Here's the drawing with two shaded views (mm, measured from the low corner). I have some questions. A direction names the side the tool comes from. Give positions to 0.01 mm unless a question says otherwise; leave off trailing zeros. Write each loop counter-clockwise with the first axis right and the second up, starting at its lowest first coordinate (ties: lowest second). Pieces come first, ordered by that corner, then holes. Notation, with made-up numbers: (53.25, -30.75) - (106.25, -30.75) arc R21 ccw to (106.25, 5.25) - close; hole circle Ø8 at (89, 46.25). An arc over 180 degrees is marked (long way). Answer as a JSON object with one key per item and string values. Group by question number.
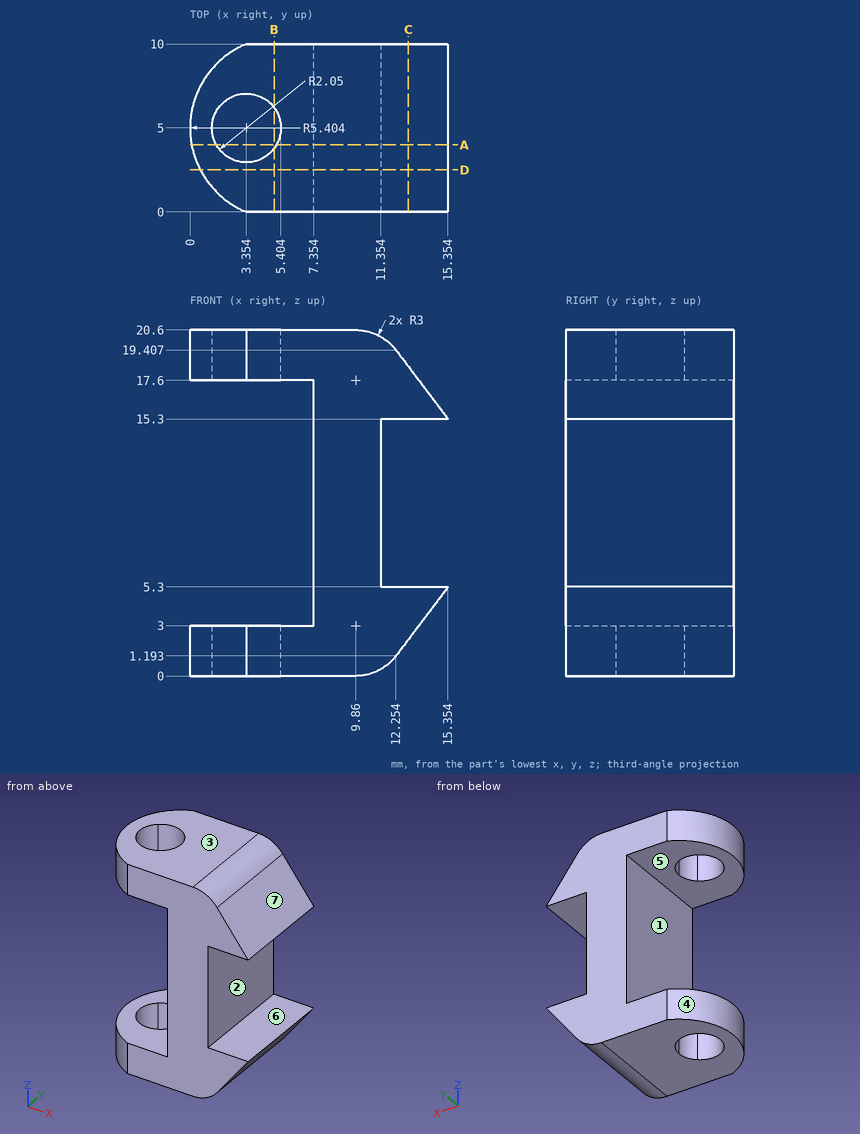
(1) I want a section at A-A, the plane y = 4. Please give me the cut outline in (x, z) (1 decimal).
(2) I want a section at C-C, the plane x = 13. Please give me the cut outline in (y, z).
(3) If we mould it in two halves opening along Z, with no side actions, what happens to the marked faces 4, 5, 6 and 7? For each: +Z half, -Z half, draft (parallel to the pull), parting line (faces both ways), or undercut.
(4) Will these pins go through, and if not, where does the flat tip stop? P1, Ø3, axis at y = 6, z = 10, coming from the +X side; P2, Ø1.2, axis at x = 13, y = 5, coming from the -Z side (1 decimal); P3, Ø3, axis at y = 7, z = 5.5, coming from the -X side.
(5) I need wall thicknesses on L1, parallel to Z at x = 2.75, y = 9; L2, parallel to Z at x = 12.75, y = 2.5; L3, parallel to Y at x = 4, z = 2.75 (1 decimal). Which ranges of each line are inside material? Lowest first, please.
(6) I want a section at B-B, the plane x = 5. Please give me the cut outline in (y, z).
(7) I want a section at D-D, the plane y = 2.5. Please give me the cut outline in (x, z) (1 decimal), and give its area (3 significant figures).
(8) For the marked faces 1, 2 and 3, which set-ups out of +Z, -Z, +X, -X, +Y, -Y let a thin tool reach every point of the face, with its end or its side?
Entries:
{
 "1": {"outline": "(0.1, 0) - (1.6, 0) - (1.6, 3) - (0.1, 3) - close; (0.1, 17.6) - (1.6, 17.6) - (1.6, 20.6) - (0.1, 20.6) - close; (5.1, 0) - (9.9, 0) arc R3 ccw to (12.3, 1.2) - (15.4, 5.3) - (11.4, 5.3) - (11.4, 15.3) - (15.4, 15.3) - (12.3, 19.4) arc R3 ccw to (9.9, 20.6) - (5.1, 20.6) - (5.1, 17.6) - (7.4, 17.6) - (7.4, 3) - (5.1, 3) - close"},
 "2": {"outline": "(0, 2.18) - (10, 2.18) - (10, 5.3) - (0, 5.3) - close; (0, 15.3) - (10, 15.3) - (10, 18.42) - (0, 18.42) - close"},
 "3": {"face 4": "draft", "face 5": "undercut", "face 6": "undercut", "face 7": "+Z half"},
 "4": {"P1": "x = 11.35", "P2": "z = 1.4", "P3": "x = 7.35"},
 "5": {"L1": "0 to 3, 17.6 to 20.6", "L2": "1.85 to 5.3, 15.3 to 18.75", "L3": "0 to 3.1, 6.9 to 10"},
 "6": {"outline": "(0, 0) - (3.78, 0) - (3.78, 3) - (0, 3) - close; (0, 17.6) - (3.78, 17.6) - (3.78, 20.6) - (0, 20.6) - close; (6.22, 0) - (10, 0) - (10, 3) - (6.22, 3) - close; (6.22, 17.6) - (10, 17.6) - (10, 20.6) - (6.22, 20.6) - close"},
 "7": {"outline": "(0.6, 0) - (9.9, 0) arc R3 ccw to (12.3, 1.2) - (15.4, 5.3) - (11.4, 5.3) - (11.4, 15.3) - (15.4, 15.3) - (12.3, 19.4) arc R3 ccw to (9.9, 20.6) - (0.6, 20.6) - (0.6, 17.6) - (7.4, 17.6) - (7.4, 3) - (0.6, 3) - close", "area": "143 mm^2"},
 "8": {"face 1": "-X, +Y, -Y", "face 2": "+X, +Y, -Y", "face 3": "+Z, +X, -X, +Y, -Y"}
}
